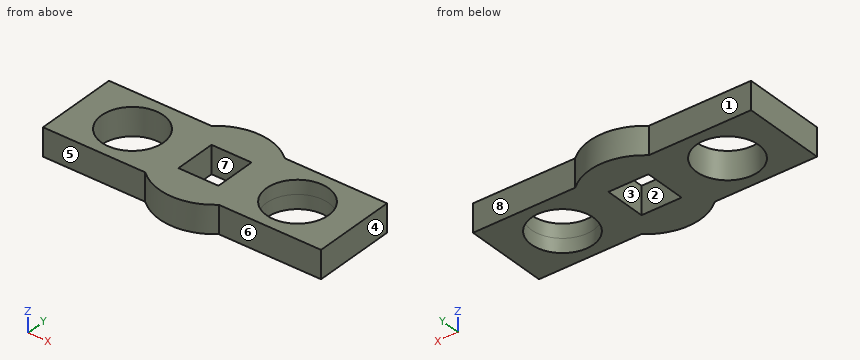
from build123d import *

# Parameters (mm, degrees)
F2_DEPTH = 1.5875
F1_W     = 4.572
F1_H     = 4.7752
F1_R     = 3.5306
F1_R_2   = 3.5344711505
F3_DEPTH = 1.5875


with BuildPart() as f2:
    # F0 (on Top) → F2 (new body, symmetric)
    with BuildSketch(Plane.XY):
        with BuildLine():
            ThreePointArc((4.2001302063, -4.7625), (5.7876302063, -2.6126302063), (6.35, 0))
            ThreePointArc((6.35, 0), (5.7876302063, 2.6126302063), (4.2001302063, 4.7625))
            Line((4.2001302063, 4.7625), (3.175, 4.7625))
            Line((3.175, 4.7625), (3.175, -4.7625))
            Line((3.175, -4.7625), (4.2001302063, -4.7625))
        make_face()
        with BuildLine():
            ThreePointArc((4.2001302063, 4.7625), (5.7876302063, 2.6126302063), (6.35, 0))
            ThreePointArc((6.35, 0), (5.7876302063, -2.6126302063), (4.2001302063, -4.7625))
            Line((4.2001302063, -4.7625), (15.875, -4.7625))
            Line((15.875, -4.7625), (15.875, 4.7625))
            Line((15.875, 4.7625), (4.2001302063, 4.7625))
        make_face()
        with BuildLine():
            Line((3.175, 4.7625), (4.2001302063, 4.7625))
            ThreePointArc((4.2001302063, 4.7625), (0, 6.35), (-4.2001302063, 4.7625))
            Line((-4.2001302063, 4.7625), (-3.175, 4.7625))
            Line((-3.175, 4.7625), (-3.175, -4.7625))
            Line((-3.175, -4.7625), (-4.2001302063, -4.7625))
            ThreePointArc((-4.2001302063, -4.7625), (0, -6.35), (4.2001302063, -4.7625))
            Line((4.2001302063, -4.7625), (3.175, -4.7625))
            Line((3.175, -4.7625), (3.175, 4.7625))
        make_face()
        with BuildLine():
            Line((-3.175, 4.7625), (-4.2001302063, 4.7625))
            ThreePointArc((-4.2001302063, 4.7625), (-6.35, 0), (-4.2001302063, -4.7625))
            Line((-4.2001302063, -4.7625), (-3.175, -4.7625))
            Line((-3.175, -4.7625), (-3.175, 4.7625))
        make_face()
        with BuildLine():
            ThreePointArc((-4.2001302063, -4.7625), (-6.35, 0), (-4.2001302063, 4.7625))
            Line((-4.2001302063, 4.7625), (-15.875, 4.7625))
            Line((-15.875, 4.7625), (-15.875, -4.7625))
            Line((-15.875, -4.7625), (-4.2001302063, -4.7625))
        make_face()
    extrude(amount=F2_DEPTH, both=True)

    # F1 (on Top) → F3 (cut, symmetric)
    with BuildSketch(Plane.XY):
        Rectangle(F1_W, F1_H)
        with Locations((9.4234, 0)):
            Circle(F1_R)
        with Locations((-9.4195288495, 0)):
            Circle(F1_R_2)
    extrude(amount=F3_DEPTH, both=True, mode=Mode.SUBTRACT)


solid = f2.part
Model file for the job. Use its own axes, mm. Face numbers are marked on the shaded views. A direction names the side the tool comes from. Coordinates: 2 decimals unless noted, no trailing zeros. Order: outer loops, then holes, each group sorted by start corner. A loop starts at its lowest first (then second) coordinate and runs counter-clockwise, first axis right, second up. Notation, with made-up numbers: (31, 18) -> (63, 18) arc R11 ccw to (63, 24) -> close; hole circle Ø7 at (71, -24.75). An arc over 180 degrees is marked (long way). Return JSON: item names as keys, results as strings. Group by question number.
Item 1: Saw through at D-D on y = -3.25. Write the cut outline in (x, z) (1 decimal).
Item 2: Tool access for the marked faces 5, 6, 7 and 8: list every direction of +Z, -Z, +X, -X, +Y, -Y with a clear straight run to the whole face (end or side of a thin tool).
Item 3: Saw through at A-A on z = 0.55. State how many separate pieces and enclosed holes the cut face has, then the cut area to 3 significant figures.
Item 4: Flat gauge pins, fed straight in: P1, Ø1, axis at x = 6, z = 0, coming from the -Y side; P2, Ø6.5, axis at x = 9.42, y = 0, coming from the +Z side (3 decimals). Where does each tip first touch, or does it go through?
Item 5: Saw through at C-C on y = 0. Write the cut outline in (x, z) (1 decimal), then the cut area to 3 significant figures.
Item 6: Pull direction X, two halves, no side cores. Call the marked faces 1, 2, 3 and 4: pulls with the +X half, pulls with the -X half, needs draft (parallel to the pull), parting line crosses it, or undercut.
Item 7: Wall check: line 1 along X through (y, z) = (-1.5, 0.8) (3 decimals); line 2 along X through (y, z) = (-0.25, 0.9) (3 decimals); line 3 along Y through (x, z) = (0, -0.4). Give the ranges that are in metal, low to high. Write a range as [from, to].
Item 8: Saw through at B-B on x = -2. Write the cut outline in (y, z).
Values found:
{
 "1": {"outline": "(-15.9, -1.6) -> (-10.8, -1.6) -> (-10.8, 1.6) -> (-15.9, 1.6) -> close; (-8, -1.6) -> (8, -1.6) -> (8, 1.6) -> (-8, 1.6) -> close; (10.8, -1.6) -> (15.9, -1.6) -> (15.9, 1.6) -> (10.8, 1.6) -> close"},
 "2": {"face 5": "+Z, -Z, -X, -Y", "face 6": "+Z, -Z, +X, -Y", "face 7": "+Z, -Z", "face 8": "+Z, -Z, +X, +Y"},
 "3": {"separate pieces": "1", "enclosed holes": "3", "area": "220 mm2"},
 "4": {"P1": "stops at y = -4.76", "P2": "passes through"},
 "5": {"outline": "(-15.9, -1.6) -> (-13, -1.6) -> (-13, 1.6) -> (-15.9, 1.6) -> close; (-5.9, -1.6) -> (-2.3, -1.6) -> (-2.3, 1.6) -> (-5.9, 1.6) -> close; (2.3, -1.6) -> (5.9, -1.6) -> (5.9, 1.6) -> (2.3, 1.6) -> close; (13, -1.6) -> (15.9, -1.6) -> (15.9, 1.6) -> (13, 1.6) -> close", "area": "41.4 mm2"},
 "6": {"face 1": "needs draft", "face 2": "undercut", "face 3": "undercut", "face 4": "pulls with the +X half"},
 "7": {"line 1": "x = [-15.875, -12.62], [-6.219, -2.286], [2.286, 6.227], [12.62, 15.875]", "line 2": "x = [-15.875, -12.945], [-5.894, -2.286], [2.286, 5.902], [12.945, 15.875]", "line 3": "y = [-6.35, -2.39], [2.39, 6.35]"},
 "8": {"outline": "(-6.03, -1.59) -> (-2.39, -1.59) -> (-2.39, 1.59) -> (-6.03, 1.59) -> close; (2.39, -1.59) -> (6.03, -1.59) -> (6.03, 1.59) -> (2.39, 1.59) -> close"}
}
